```python
from build123d import *

# Parameters (mm, degrees)
SKETCH1_R           = 3.1115
SKETCH1_R_2         = 2.9845
BOSS_EXTRUDE1_DEPTH = 1.905
CUT_EXTRUDE1_DEPTH  = 1.651
BOSS_EXTRUDE2_DEPTH = 1.27
FILLET4_R           = 0.762


with BuildPart() as part:
    # Sketch1 → Boss-Extrude1 (new body)
    with BuildSketch(Plane.XY):
        with BuildLine():
            Line((61.17139063, 26.332220791), (60.704944856, 11.966179777))
            ThreePointArc((60.704944856, 11.966179777), (55.469656343, 7.945478091), (52.551985386, 13.866751944))
            ThreePointArc((52.551985386, 13.866751944), (53.150243594, 19.068304512), (52.551985386, 24.269857079))
            ThreePointArc((52.551985386, 24.269857079), (49.685224569, 38.006015424), (49.090889591, 52.025542148))
            ThreePointArc((49.090889591, 52.025542148), (51.146965053, 52.083276575), (52.012792223, 53.949053326))
            ThreePointArc((52.012792223, 53.949053326), (52.29374244, 55.401070195), (52.012792223, 56.853087065))
            ThreePointArc((52.012792223, 56.853087065), (51.509420049, 58.711680371), (49.661768019, 58.169523016))
            Line((49.661768019, 58.169523016), (50.574786632, 66.4382933))
            Line((50.574786632, 66.4382933), (52.012792223, 66.4382933))
            ThreePointArc((52.012792223, 66.4382933), (52.772258586, 66.349188863), (53.373853233, 66.821219197))
            Line((53.373853233, 66.821219197), (53.909482304, 67.76887063))
            Line((53.909482304, 67.76887063), (57.57460461, 68.813123354))
            ThreePointArc((57.57460461, 68.813123354), (59.75855859, 68.176663617), (60.704944856, 66.10806771))
            Line((60.704944856, 66.10806771), (60.704944856, 59.081610081))
            Line((60.704944856, 59.081610081), (61.617031921, 58.169523016))
            Line((61.617031921, 58.169523016), (61.617031921, 54.655997897))
            Line((61.617031921, 54.655997897), (58.390036251, 52.025542148))
            Line((58.390036251, 52.025542148), (58.390036251, 44.445572853))
            Line((58.390036251, 44.445572853), (61.617031921, 40.486752766))
            Line((61.617031921, 40.486752766), (61.819220674, 27.533280913))
            Line((61.819220674, 27.533280913), (61.17139063, 26.332220791))
        make_face()
        with Locations((56.438703811, 64.020773394)):
            Circle(SKETCH1_R, mode=Mode.SUBTRACT)
        with Locations((56.241951704, 11.95715462)):
            Circle(SKETCH1_R_2, mode=Mode.SUBTRACT)
    extrude(amount=BOSS_EXTRUDE1_DEPTH)

    # Sketch2 → Cut-Extrude1 (cut)
    with BuildSketch(Plane.XY.offset(1.905)):
        with BuildLine():
            Line((60.704944856, 59.081610081), (61.160988389, 58.625566549))
            ThreePointArc((61.160988389, 58.625566549), (58.418398779, 55.641187467), (56.855649817, 51.901383735))
            ThreePointArc((56.855649817, 51.901383735), (57.672831025, 39.378266905), (61.819220674, 27.533280913))
            Line((61.819220674, 27.533280913), (61.17139063, 26.332220791))
            ThreePointArc((61.17139063, 26.332220791), (56.696533643, 38.574284868), (55.8334865, 51.57996161))
            ThreePointArc((55.8334865, 51.57996161), (57.423428617, 55.880027317), (60.704944856, 59.081610081))
        make_face()
    extrude(amount=-CUT_EXTRUDE1_DEPTH, mode=Mode.SUBTRACT)

    # Sketch3 → Boss-Extrude2 (add)
    with BuildSketch(Plane.XY.offset(1.905)):
        with BuildLine():
            Line((61.819220674, 27.533280913), (61.617031921, 40.486752766))
            Line((61.617031921, 40.486752766), (58.390036251, 44.445572853))
            Line((58.390036251, 44.445572853), (58.390036251, 52.025542148))
            Line((58.390036251, 52.025542148), (61.617031921, 54.655997897))
            Line((61.617031921, 54.655997897), (61.617031921, 58.169523016))
            Line((61.617031921, 58.169523016), (61.160988389, 58.625566549))
            ThreePointArc((61.160988389, 58.625566549), (58.418398779, 55.641187467), (56.855649817, 51.901383735))
            ThreePointArc((56.855649817, 51.901383735), (57.672831025, 39.378266905), (61.819220674, 27.533280913))
        make_face()
    extrude(amount=BOSS_EXTRUDE2_DEPTH)

    # Fillet4
    fillet4_edges = [part.edges().sort_by_distance(p)[0] for p in [
        (50.574786632, 66.4382933, 0.9525),
    ]]
    fillet(fillet4_edges, radius=FILLET4_R)


solid = part.part
```
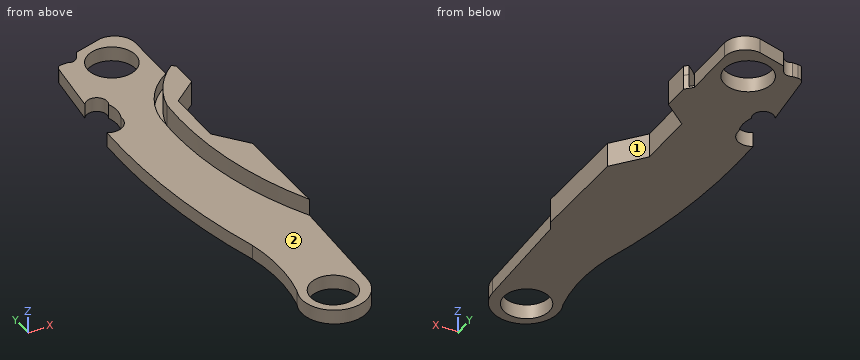
CAD build for the part. Positions are in the model's coordinates, mm. Face numbers are marked on the shaded views. Coordinates: 2 decimals unless noted, no trailing zeros. Order: outer loops, then holes, each group sorted by start corner. A loop starts at its lowest first (then second) coordinate and runs counter-clockwise, first axis right, second up.
(1) Mould opens along Y. For the marked faces 1 and 2 say: released by +Y, released by -Y, zero draft, split by the parting line, or undercut.
Solution:
face 1: undercut
face 2: zero draft
(2) Saw through at D-D, the plane y = 21.5. Write the cut outline in (x, z) (1 decimal), and give its area (3 significant figures).
Solution:
outline: (53, 0) - (61, 0) - (61, 1.9) - (53, 1.9) - close
area: 15.2 mm2
(3) Saw through at B-B, the plane y = 37.5. Write the cut outline in (x, z) (3 decimals), and give its area (3 significant figures).
Solution:
outline: (49.75, 0) - (61.664, 0) - (61.664, 3.175) - (58.096, 3.175) - (58.096, 0.254) - (56.937, 0.254) - (56.937, 1.905) - (49.75, 1.905) - close
area: 25.3 mm2
(4) Pin check, flat tips, straight feed: pin 1 Ø5.5 at (x, y) = (56.24, 11.96) entering from +Z; pin 2 Ø3 at (x, y) = (54, 42) entering from -Z; pin 3 Ø0.6 at (x, z) = (51.5, 1) entering from +Y; pin 4 Ø1 at (y, z) = (61.5, 1) entering from +X. Stop position of each tip, or through.
Solution:
pin 1: passes through
pin 2: stops at z = 0
pin 3: stops at y = 66.44
pin 4: stops at x = 60.7
(5) Drill centre lines: L1, parallel to Y at x = 60.25, z = 0.4; L2, parallel to Y at x = 53.75, z = 0.4; L3, parallel to Z at x = 53, y = 45.5 (3 decimals). Where is each one in solid material? Low to high.
Solution:
L1: y = 10.18 to 28.14, 30.94 to 42.16, 53.54 to 57.85, 58.79 to 67.62
L2: y = 8.79 to 10.31, 13.6 to 62.45, 65.59 to 67.49
L3: z = 0 to 1.905
(6) Saw through at A-A, the plane z = 1.1. Write the cut outline in (x, y), and give its area (3 significant figures).
Solution:
outline: (49.09, 52.03) arc R85.98 ccw to (52.55, 24.27) arc R22.91 cw to (52.55, 13.87) arc R4.27 ccw (long way) to (60.7, 11.97) - (61.17, 26.33) arc R46.02 cw to (55.83, 51.58) arc R10.42 cw to (60.7, 59.08) - (60.7, 66.11) arc R2.73 ccw to (57.57, 68.81) - (53.91, 67.77) - (53.37, 66.82) arc R1 cw to (52.01, 66.44) - (51.26, 66.44) arc R0.76 ccw to (50.5, 65.76) - (49.66, 58.17) arc R1.35 cw (long way) to (52.01, 56.85) arc R3.89 cw to (52.01, 53.95) arc R1.95 cw to start; (56.86, 51.9) arc R46.36 ccw to (61.82, 27.53) - (61.62, 40.49) - (58.39, 44.45) - (58.39, 52.03) - (61.62, 54.66) - (61.62, 58.17) - (61.16, 58.63) arc R11.73 ccw to start; hole circle Ø5.97 at (56.24, 11.96); hole circle Ø6.22 at (56.44, 64.02)
area: 476 mm2
(7) Saw through at C-C, the plane y = 47. Write the cut outline in (x, z) (3 decimals), and give its area (3 significant figures).
Solution:
outline: (49.04, 0) - (58.39, 0) - (58.39, 3.175) - (56.769, 3.175) - (56.769, 0.254) - (55.714, 0.254) - (55.714, 1.905) - (49.04, 1.905) - close
area: 18.1 mm2
